Could you check a few things on this model? Use its own coordinates, in mm. Face numbers are marked on the shaded views. A direction names the side the tool comes from. Give positions to 0.01 mm unless a question says otherwise; leave off trailing zeros. Write each loop counter-clockwise with the first axis right and the second up, starting at its lowest first coordinate (ties: lowest second). Pieces come first, ordered by that corner, then holes. Notation, with made-up numbers: M -1.75,-35.75 L 12.25,-35.75 A21 ccw 12.25,-10.75 Z; hole C 11,36.5 d10. An arc over 180 degrees is marked long. Use one line per item in the form item = value.
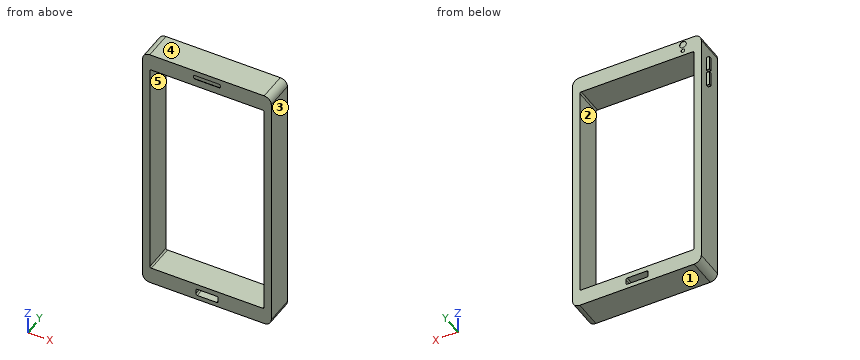
from build123d import *

# Parameters (mm, degrees)
F1_DEPTH = 19.05
F2_W     = 2.54
F2_H     = 12.7
F3_DEPTH = 2.54
F4_DEPTH = 25.4
F5_DEPTH = 25.4
F7_DEPTH = 0.254
F8_R     = 2.995029
F8_R_2   = 1.619254
F9_DEPTH = 0.254


with BuildPart() as f1:
    # F0 (on Front) → F1 (new body)
    with BuildSketch(Plane.XZ):
        with BuildLine():
            Line((50.8, 114.3), (-50.8, 114.3))
            ThreePointArc((-50.8, 114.3), (-55.290128, 112.440128), (-57.15, 107.95))
            Line((-57.15, 107.95), (-57.15, -107.95))
            ThreePointArc((-57.15, -107.95), (-55.290128, -112.440128), (-50.8, -114.3))
            Line((-50.8, -114.3), (50.8, -114.3))
            ThreePointArc((50.8, -114.3), (55.290128, -112.440128), (57.15, -107.95))
            Line((57.15, -107.95), (57.15, 107.95))
            ThreePointArc((57.15, 107.95), (55.290128, 112.440128), (50.8, 114.3))
        make_face()
        with BuildLine():
            ThreePointArc((-9.873155, -105.40096), (-9.492607, -104.482236), (-8.573882, -104.101688))
            Line((-8.573882, -104.101688), (8.573882, -104.101688))
            ThreePointArc((8.573882, -104.101688), (9.492607, -104.482236), (9.873155, -105.40096))
            Line((9.873155, -105.40096), (9.873155, -108.98943))
            ThreePointArc((9.873155, -108.98943), (9.492607, -109.908154), (8.573882, -110.288702))
            Line((8.573882, -110.288702), (-8.573882, -110.288702))
            ThreePointArc((-8.573882, -110.288702), (-9.492607, -109.908154), (-9.873155, -108.98943))
            Line((-9.873155, -108.98943), (-9.873155, -105.40096))
        make_face(mode=Mode.SUBTRACT)
        with BuildLine():
            ThreePointArc((-50.673, 98.178406), (-50.292452, 99.09713), (-49.373728, 99.477679))
            Line((-49.373728, 99.477679), (49.373728, 99.477679))
            ThreePointArc((49.373728, 99.477679), (50.292452, 99.09713), (50.673, 98.178406))
            Line((50.673, 98.178406), (50.673, -98.178406))
            ThreePointArc((50.673, -98.178406), (50.292452, -99.09713), (49.373728, -99.477679))
            Line((49.373728, -99.477679), (-49.373728, -99.477679))
            ThreePointArc((-49.373728, -99.477679), (-50.292452, -99.09713), (-50.673, -98.178406))
            Line((-50.673, -98.178406), (-50.673, 98.178406))
        make_face(mode=Mode.SUBTRACT)
    extrude(amount=F1_DEPTH)

    # F2 (on face) → F3 (join)
    with BuildSketch(Plane(origin=(-57.15, 0, 0), x_dir=(0, -1, 0), z_dir=(-1, 0, 0))):
        with Locations((9.525, 90.329596)):
            Rectangle(F2_W, F2_H)
        with Locations((9.525, 75.089596)):
            Rectangle(F2_W, F2_H)
    extrude(amount=F3_DEPTH)

    # F0 (on Front) → F4 (join)
    with BuildSketch(Plane.XZ):
        with BuildLine():
            Line((50.8, 114.3), (-50.8, 114.3))
            ThreePointArc((-50.8, 114.3), (-55.290128, 112.440128), (-57.15, 107.95))
            Line((-57.15, 107.95), (-57.15, -107.95))
            ThreePointArc((-57.15, -107.95), (-55.290128, -112.440128), (-50.8, -114.3))
            Line((-50.8, -114.3), (50.8, -114.3))
            ThreePointArc((50.8, -114.3), (55.290128, -112.440128), (57.15, -107.95))
            Line((57.15, -107.95), (57.15, 107.95))
            ThreePointArc((57.15, 107.95), (55.290128, 112.440128), (50.8, 114.3))
        make_face()
        with BuildLine():
            ThreePointArc((-9.873155, -105.40096), (-9.492607, -104.482236), (-8.573882, -104.101688))
            Line((-8.573882, -104.101688), (8.573882, -104.101688))
            ThreePointArc((8.573882, -104.101688), (9.492607, -104.482236), (9.873155, -105.40096))
            Line((9.873155, -105.40096), (9.873155, -108.98943))
            ThreePointArc((9.873155, -108.98943), (9.492607, -109.908154), (8.573882, -110.288702))
            Line((8.573882, -110.288702), (-8.573882, -110.288702))
            ThreePointArc((-8.573882, -110.288702), (-9.492607, -109.908154), (-9.873155, -108.98943))
            Line((-9.873155, -108.98943), (-9.873155, -105.40096))
        make_face(mode=Mode.SUBTRACT)
        with BuildLine():
            ThreePointArc((-50.673, 98.178406), (-50.292452, 99.09713), (-49.373728, 99.477679))
            Line((-49.373728, 99.477679), (49.373728, 99.477679))
            ThreePointArc((49.373728, 99.477679), (50.292452, 99.09713), (50.673, 98.178406))
            Line((50.673, 98.178406), (50.673, -98.178406))
            ThreePointArc((50.673, -98.178406), (50.292452, -99.09713), (49.373728, -99.477679))
            Line((49.373728, -99.477679), (-49.373728, -99.477679))
            ThreePointArc((-49.373728, -99.477679), (-50.292452, -99.09713), (-50.673, -98.178406))
            Line((-50.673, -98.178406), (-50.673, 98.178406))
        make_face(mode=Mode.SUBTRACT)
    extrude(amount=F4_DEPTH)

    # F0 (on Front) → F5 (join)
    with BuildSketch(Plane.XZ):
        with BuildLine():
            Line((50.8, 114.3), (-50.8, 114.3))
            ThreePointArc((-50.8, 114.3), (-55.290128, 112.440128), (-57.15, 107.95))
            Line((-57.15, 107.95), (-57.15, -107.95))
            ThreePointArc((-57.15, -107.95), (-55.290128, -112.440128), (-50.8, -114.3))
            Line((-50.8, -114.3), (50.8, -114.3))
            ThreePointArc((50.8, -114.3), (55.290128, -112.440128), (57.15, -107.95))
            Line((57.15, -107.95), (57.15, 107.95))
            ThreePointArc((57.15, 107.95), (55.290128, 112.440128), (50.8, 114.3))
        make_face()
        with BuildLine():
            ThreePointArc((-9.873155, -105.40096), (-9.492607, -104.482236), (-8.573882, -104.101688))
            Line((-8.573882, -104.101688), (8.573882, -104.101688))
            ThreePointArc((8.573882, -104.101688), (9.492607, -104.482236), (9.873155, -105.40096))
            Line((9.873155, -105.40096), (9.873155, -108.98943))
            ThreePointArc((9.873155, -108.98943), (9.492607, -109.908154), (8.573882, -110.288702))
            Line((8.573882, -110.288702), (-8.573882, -110.288702))
            ThreePointArc((-8.573882, -110.288702), (-9.492607, -109.908154), (-9.873155, -108.98943))
            Line((-9.873155, -108.98943), (-9.873155, -105.40096))
        make_face(mode=Mode.SUBTRACT)
        with BuildLine():
            ThreePointArc((-50.673, 98.178406), (-50.292452, 99.09713), (-49.373728, 99.477679))
            Line((-49.373728, 99.477679), (49.373728, 99.477679))
            ThreePointArc((49.373728, 99.477679), (50.292452, 99.09713), (50.673, 98.178406))
            Line((50.673, 98.178406), (50.673, -98.178406))
            ThreePointArc((50.673, -98.178406), (50.292452, -99.09713), (49.373728, -99.477679))
            Line((49.373728, -99.477679), (-49.373728, -99.477679))
            ThreePointArc((-49.373728, -99.477679), (-50.292452, -99.09713), (-50.673, -98.178406))
            Line((-50.673, -98.178406), (-50.673, 98.178406))
        make_face(mode=Mode.SUBTRACT)
    extrude(amount=F5_DEPTH)

    # F6 (on face) → F7 (cut)
    with BuildSketch(Plane.XZ.offset(25.4)):
        with BuildLine():
            ThreePointArc((-12.027082, 107.484314), (-11.646534, 106.565589), (-10.72781, 106.185041))
            Line((-10.72781, 106.185041), (10.72781, 106.185041))
            ThreePointArc((10.72781, 106.185041), (11.646534, 106.565589), (12.027082, 107.484314))
            Line((12.027082, 107.484314), (12.027082, 108.415686))
            ThreePointArc((12.027082, 108.415686), (11.646534, 109.334411), (10.72781, 109.714959))
            Line((10.72781, 109.714959), (-10.72781, 109.714959))
            ThreePointArc((-10.72781, 109.714959), (-11.646534, 109.334411), (-12.027082, 108.415686))
            Line((-12.027082, 108.415686), (-12.027082, 107.484314))
        make_face()
    extrude(amount=-F7_DEPTH, mode=Mode.SUBTRACT)

    # F8 (on face) → F9 (cut)
    with BuildSketch(Plane.XZ):
        with Locations((-40.86072, 110.174194)):
            Circle(F8_R)
        with Locations((-40.86072, 104.160182)):
            Circle(F8_R_2)
    extrude(amount=F9_DEPTH, mode=Mode.SUBTRACT)


solid = f1.part
1) I want a section at A-A, the plane x = 0.5. Please give me the cut outline in (y, z).
Checked values:
outline = M -25.4,-114.3 L 0,-114.3 L 0,-110.29 L -25.4,-110.29 Z; M -25.4,-104.1 L 0,-104.1 L 0,-99.48 L -25.4,-99.48 Z; M -25.4,99.48 L 0,99.48 L 0,114.3 L -25.4,114.3 L -25.4,109.71 L -25.15,109.71 L -25.15,106.19 L -25.4,106.19 Z
2) If I drill on L1, parallel to Z at x = 2, y = -7; L2, parallel to X at y = -5.75, z = 11; L3, parallel to Z at x = -48, y = -12.5, over which ranges is the centre line in solid material (lowest first)?
Checked values:
L1 = -114.3 to -110.29, -104.1 to -99.48, 99.48 to 114.3
L2 = -57.15 to -50.67, 50.67 to 57.15
L3 = -114.3 to -99.48, 99.48 to 114.3
3) For the marked faces 4 and 5, which set-ups out of +Z, -Z, +X, -X, +Y, -Y let a thin tool reach every point of the face, with its end or its side?
Checked values:
face_4 = +Z, +X, -X, +Y, -Y
face_5 = +Y, -Y
4) For pin 1 Ø6 at (y, z) = (-16.5, 5.5) entering from -X; pin 2 Ø0.8 at (x, y) = (-58.5, -10) entering from +Z; pin 3 Ø1.9 at (x, z) = (-40.86, 104.16) entering from +Y; pin 4 Ø10 at (x, z) = (44.5, -71.5) entering from -Y, each with a flat end and sliding along its axis, tell me the tip position at first contact or that it passes through.
Checked values:
pin_1 = -57.15
pin_2 = 96.68
pin_3 = -0.25
pin_4 = through
5) I want a section at B-B, the plane z = 88.5. Please give me the cut outline in (x, y) (3 decimals), plus the area to 3 significant figures.
Checked values:
outline = M -59.69,-10.795 L -57.15,-10.795 L -57.15,-25.4 L -50.673,-25.4 L -50.673,0 L -57.15,0 L -57.15,-8.255 L -59.69,-8.255 Z; M 50.673,-25.4 L 57.15,-25.4 L 57.15,0 L 50.673,0 Z
area = 335 mm2
6) Thinking about a two-plate mould opening in X: for the marked faces 1, 2 and 3, which applies, released by +X, released by -X, zero draft, split by the parting line, or undercut?
Checked values:
face_1 = zero draft
face_2 = undercut
face_3 = released by +X
7) I want a section at C-C, the plane y = -6. Please give me the cut outline in (x, z).
Checked values:
outline = M -57.15,-107.95 A6.35 ccw -50.8,-114.3 L 50.8,-114.3 A6.35 ccw 57.15,-107.95 L 57.15,107.95 A6.35 ccw 50.8,114.3 L -50.8,114.3 A6.35 ccw -57.15,107.95 Z; hole M -50.67,-98.18 A1.3 ccw -49.37,-99.48 L 49.37,-99.48 A1.3 ccw 50.67,-98.18 L 50.67,98.18 A1.3 ccw 49.37,99.48 L -49.37,99.48 A1.3 ccw -50.67,98.18 Z; hole M -9.87,-108.99 A1.3 ccw -8.57,-110.29 L 8.57,-110.29 A1.3 ccw 9.87,-108.99 L 9.87,-105.4 A1.3 ccw 8.57,-104.1 L -8.57,-104.1 A1.3 ccw -9.87,-105.4 Z
8) I want a section at D-D, the plane x = -46. Please give me the cut outline in (y, z), plus the area to 3 significant figures.
Checked values:
outline = M -25.4,-114.3 L 0,-114.3 L 0,-99.48 L -25.4,-99.48 Z; M -25.4,99.48 L 0,99.48 L 0,114.3 L -25.4,114.3 Z
area = 753 mm2
